```python
from build123d import *

# Parameters (mm, degrees)
CHANFREIN1_SIZE              = 1
ESQUISSE3_R                  = 6
ENL_V_MAT_EXTRU_2_DEPTH      = 146
ENL_V_MAT_EXTRU_1_DEPTH      = 146
R_P_TITION_CIRCULAIRE1_COUNT = 4
CHANFREIN2_SIZE              = 1
CHANFREIN2_SIZE2             = 1.732050808


with BuildPart() as part:
    # Esquisse1 → Révolution1 (revolve)
    with BuildSketch(Plane(origin=(0, 0, 0), x_dir=(0, 0, -1), z_dir=(1, 0, 0)), mode=Mode.PRIVATE) as r_volution1_sk:
        Polygon((-145, 0), (-145, 10), (-125, 10), (-125, 12.5), (-10, 12.5), (-10, 22.5), (0, 22.5), (0, 0), align=None)
    revolve(r_volution1_sk.sketch.rotate(Axis((0, 0, 0), (0, 0, 1)), 90), axis=Axis((0, 0, 0), (0, 0, 1)))  # turned: the seam where the file's is

    # Chanfrein1
    chanfrein1_edges = [part.edges().sort_by_distance(p)[0] for p in [
        (22.5, 0, 0),
        (22.5, 0, 10),
        (10, 0, 145),
    ]]
    chamfer(chanfrein1_edges, length=CHANFREIN1_SIZE)

    # Esquisse3 → Enlèv. mat.-Extru.2 (cut, through all)
    with BuildSketch(Plane(origin=(0, 0, 0), x_dir=(-1, 0, 0), z_dir=(0, 0, -1))):
        Circle(ESQUISSE3_R)
    extrude(amount=-ENL_V_MAT_EXTRU_2_DEPTH, mode=Mode.SUBTRACT)

    # Esquisse2 → Enlèv. mat.-Extru.1 (cut, through all)
    with BuildSketch(Plane(origin=(0, 0, 0), x_dir=(-1, 0, 0), z_dir=(0, 0, -1))):
        with BuildLine():
            Line((-3.1, 22.285421243), (-3.1, 17))
            Line((-3.1, 17), (3.1, 17))
            Line((3.1, 17), (3.1, 22.285421243))
            ThreePointArc((3.1, 22.285421243), (0, 22.5), (-3.1, 22.285421243))
        make_face()
    enl_v_mat_extru_1 = extrude(amount=-ENL_V_MAT_EXTRU_1_DEPTH, mode=Mode.SUBTRACT)

    # Répétition circulaire1: Enlèv. mat.-Extru.1 ×4 about axis
    r_p_tition_circulaire1_axis = Axis((0, 0, 0), (0, 0, 1))
    for i in range(1, R_P_TITION_CIRCULAIRE1_COUNT):
        add(enl_v_mat_extru_1.rotate(r_p_tition_circulaire1_axis, i * 360 / R_P_TITION_CIRCULAIRE1_COUNT), mode=Mode.SUBTRACT)

    # Chanfrein2
    chanfrein2_edges = [part.edges().sort_by_distance(p)[0] for p in [
        (12.5, 0, 125),
    ]]
    chanfrein2_side = [part.faces().sort_by_distance(p)[0] for p in [
        (10.353553391, 0, 125),
    ]]
    chamfer(chanfrein2_edges, length=CHANFREIN2_SIZE, length2=CHANFREIN2_SIZE2, reference=chanfrein2_side[0])


solid = part.part
```
Read the model definition and answer for the solid it produces. Units are mm, in the model's axes. A direction names the side the tool comes from. Give positions to 0.01 mm unless a question says otherwise; leave off trailing zeros. Order: outer loops, then holes, each group sorted by start corner. A loop starts at its lowest first (then second) coordinate and runs counter-clockwise, first axis right, second up.
(1) For faces 4 (the flat face through (0, 17, 5)), 5 (the flat face through (-20, -3.1, 5)), 6 (the cylindrical face through (10, 0, 134)), determine the directions among +Z, -Z, +X, -X, +Y, -Y from which every point of the face is accessible in a straight line to the end or side of a thin tool.
(2) Straight lines are drawn through the part: L1, parallel to Y at x = 0, z = 59.5; L2, parallel to Z at x = 17, y = 8; L3, parallel to Z at x = 8, y = 8. For each, find the intervals that lie inside material, in ascending order.
(3) For a pull along X with two mould halves and no side action, classify faces 1 (the flat face through (3.1, -20, 5)), 2 (the flat face through (20, -3.1, 5)), 3 (the conical face through (-15.45, -15.18, 0.16)) as released by +X, released by -X, zero draft, split by the parting line, or undercut.
(4) Find section D-D (z = 126.5). Give the vertices of the cut face in (x, y).
(5) Find section A-A (x = 0). Give the vertices of the cut face in (y, z), plus the area to 3 significant figures.
(6) Given pin 1 (1.9 mm diameter, centred on y = 1.5, z = 4.5, fed in from -X); pin 2 (1 mm diameter, centred on x = -15.5, y = -5.5, fed in from +Z); pin 3 (1.6 mm diameter, centred on x = 20.5, z = 7.5, fed in from -Y), each flat-ended and moving along its own axis, determine where each tip first touches the part or whether it passes through.
(7) Find section C-C (z = 87). Give the vertices of the cut face in (x, y).
Result sheet:
1. face 4: +Z, -Z, +Y
1. face 5: +Z, -Z, -X
1. face 6: +Z
2. L1: y = -12.5 to -6, 6 to 12.5
2. L2: z = 0 to 10
2. L3: z = 0 to 125
3. face 1: undercut
3. face 2: zero draft
3. face 3: released by -X
4. outline: circle Ø20 at (0, 0); hole circle Ø12 at (0, 0)
5. outline: (-17, 0) - (-6, 0) - (-6, 145) - (-9, 145) - (-10, 144) - (-10, 125) - (-11.5, 125) - (-12.5, 123.27) - (-12.5, 10) - (-17, 10) - close; (6, 0) - (17, 0) - (17, 10) - (12.5, 10) - (12.5, 123.27) - (11.5, 125) - (10, 125) - (10, 144) - (9, 145) - (6, 145) - close
5. area: 1,870 mm2
6. pin 1: stops at x = -17
6. pin 2: stops at z = 10
6. pin 3: stops at y = -10.87
7. outline: circle Ø25 at (0, 0); hole circle Ø12 at (0, 0)
